Can you work these out from the drawing? Everything is in mm from the part's minimum corner. Give positions to 0.01 mm unless a question says otherwise; leave off trailing zeros. Loops run counter-clockwise (first coordinate to the right, second up) from the corner with the lowest first, then second, coordinate; pieces in that order, holes last. Notation, with made-up numbers: (32.25, 89) -> (82.25, 89) arc R28 ccw to (82.25, 128) -> close; hole circle Ø3 at (-24.5, 1.25). An arc over 180 degrees is marked (long way). Return JSON: item names as keys, results as strings. Group by question number.
Q1. Thinking about a two-plate mould opening in X: for the marked faces 1, 2 and 3, which applies, pulls with the +X half, pulls with the -X half, needs draft (parallel to the pull), parting line crosses it, or undercut?
Q2. I need wall thicknesses on line 1 along X through (y, z) = (48.5, 32); line 2 along Y through (x, z) = (38, 20); line 3 along Z through (x, y) = (17, 39.5). Which ranges of each line are inside material? Lowest first, please. Write a range as [from, to].
Q3. Will these pins go through, and if not, where does the flat tip stop? pin 1 (4 mm diameter, centred on x = 44.5, y = 30, fed in from +Z); pin 2 (12 mm diameter, centred on x = 46, z = 38.5, fed in from +Y); pin 3 (2 mm diameter, centred on y = 27.5, z = 15, fed in from -X).
Q4. Suppose I cut it at B-B, the plane z = 32. Please give me the cut outline in (x, y), and give its area (3 significant figures).
Q5. Suppose I cut it at C-C, the plane y = 14. Please give me the cut outline in (x, z).
Q6. Suppose I cut it at A-A, the plane x = 32. Please give me the cut outline in (y, z), and give its area (3 significant figures).
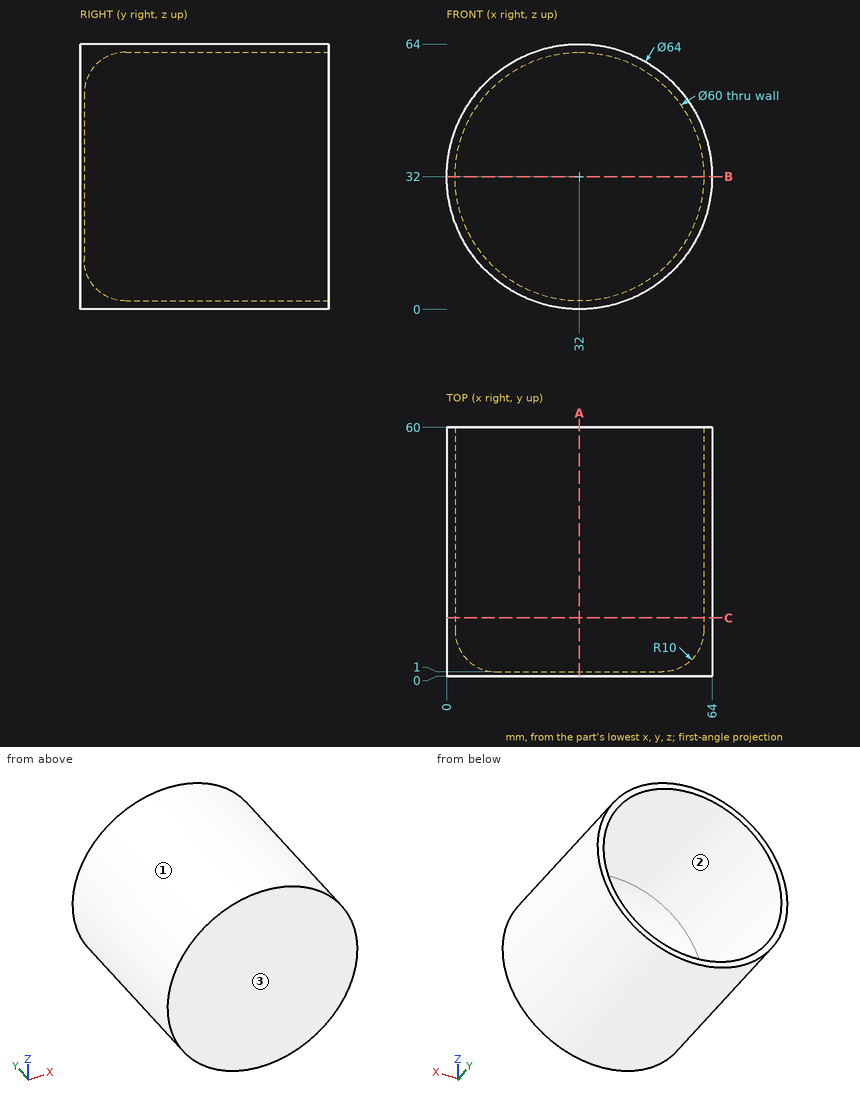
Ans:
{
 "1": {"face 1": "parting line crosses it", "face 2": "undercut", "face 3": "needs draft"},
 "2": {"line 1": "x = [0, 2], [62, 64]", "line 2": "y = [0, 1]", "line 3": "z = [3.73, 6.02], [57.98, 60.27]"},
 "3": {"pin 1": "stops at z = 62.23", "pin 2": "stops at y = 1.1", "pin 3": "stops at x = 4.29"},
 "4": {"outline": "(0, 0) -> (64, 0) -> (64, 60) -> (62, 60) -> (62, 11) arc R10 cw to (52, 1) -> (12, 1) arc R10 cw to (2, 11) -> (2, 60) -> (0, 60) -> close", "area": "343 mm^2"},
 "5": {"outline": "circle Ø64 at (32, 32); hole circle Ø60 at (32, 32)"},
 "6": {"outline": "(0, 0) -> (60, 0) -> (60, 2) -> (11, 2) arc R10 cw to (1, 12) -> (1, 52) arc R10 cw to (11, 62) -> (60, 62) -> (60, 64) -> (0, 64) -> close", "area": "343 mm^2"}
}
